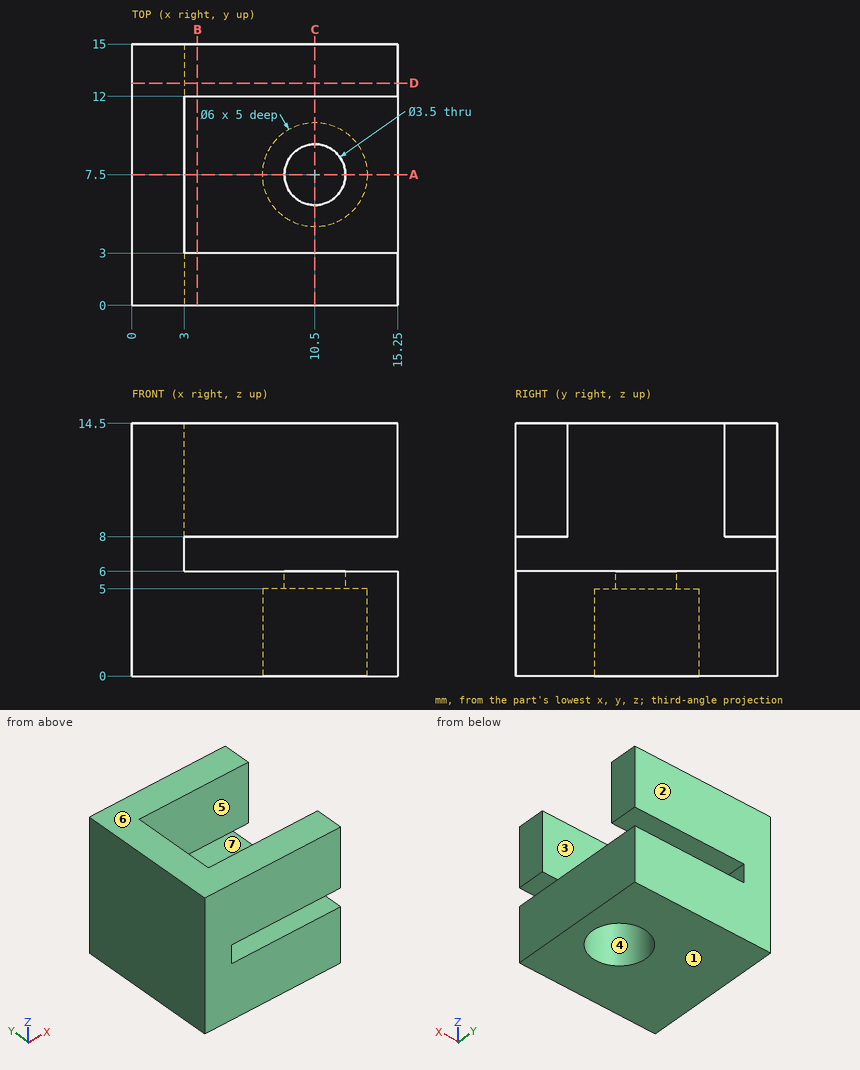
The drawing under review shows one solid part. Ordinate dimensions are in mm from its lowest x, y, z. A direction names the side the tool comes from. Coordinates: 2 decimals unless noted, no trailing zeros. Order: outer loops, then holes, each group sorted by start corner. A loop starts at its lowest first (then second) coordinate and runs counter-clockwise, first axis right, second up. Notation, with made-up numbers: (-17, 17.5) -> (35, 17.5) arc R26 ccw to (35, 32.5) -> close; hole circle Ø7 at (83.25, 85.5). An arc over 180 degrees is marked (long way). Return JSON: item names as keys, results as strings.
1. We need section A-A on y = 7.5. Write out the cut boundary in (x, z), and give its area (3 significant figures).
Answer block:
{"outline": "(0, 0) -> (7.5, 0) -> (7.5, 5) -> (8.75, 5) -> (8.75, 6) -> (3, 6) -> (3, 14.5) -> (0, 14.5) -> close; (12.25, 5) -> (13.5, 5) -> (13.5, 0) -> (15.25, 0) -> (15.25, 6) -> (12.25, 6) -> close", "area": "83.5 mm²"}
2. We need section D-D on y = 12.75. Write out the cut boundary in (x, z), and give its area (3 significant figures).
Answer block:
{"outline": "(0, 0) -> (15.25, 0) -> (15.25, 6) -> (3, 6) -> (3, 8) -> (15.25, 8) -> (15.25, 14.5) -> (0, 14.5) -> close", "area": "197 mm²"}
3. Machinability: for the marked faces 5, 6 and 7, which of the approach directions +Z, -Z, +X, -X, +Y, -Y give a long, thin tool a straight path to every point of the face, cutting with its end or side? Answer none if there is none.
Answer block:
{"face 5": "+Z, +X", "face 6": "+Z, +X, -X, +Y, -Y", "face 7": "+X, +Y, -Y"}
4. For pin 1 Ø5 at (x, y) = (5, 4) entering from -Z; pin 2 Ø7 at (x, y) = (10.5, 7.5) entering from +Z; pin 3 Ø2.5 at (y, z) = (6.5, 10) entering from +X, all flat-tipped, find the tip position at first contact; note any pin that passes through.
Answer block:
{"pin 1": "z = 0", "pin 2": "z = 6", "pin 3": "x = 3"}
5. The part is to be moulded in two halves that separate along Y. For the marked faces 1, 2, 3 and 4, say which applies: +Y half, -Y half, draft (parallel to the pull), parting line (faces both ways), or undercut.
Answer block:
{"face 1": "draft", "face 2": "+Y half", "face 3": "undercut", "face 4": "undercut"}
6. We need section B-B on x = 3.75. Write out the cut boundary in (y, z), and give its area (3 significant figures).
Answer block:
{"outline": "(0, 0) -> (15, 0) -> (15, 6) -> (0, 6) -> close; (0, 8) -> (3, 8) -> (3, 14.5) -> (0, 14.5) -> close; (12, 8) -> (15, 8) -> (15, 14.5) -> (12, 14.5) -> close", "area": "129 mm²"}
7. We need section C-C on x = 10.5. Write out the cut boundary in (y, z), and give its area (3 significant figures).
Answer block:
{"outline": "(0, 0) -> (4.5, 0) -> (4.5, 5) -> (5.75, 5) -> (5.75, 6) -> (0, 6) -> close; (0, 8) -> (3, 8) -> (3, 14.5) -> (0, 14.5) -> close; (9.25, 5) -> (10.5, 5) -> (10.5, 0) -> (15, 0) -> (15, 6) -> (9.25, 6) -> close; (12, 8) -> (15, 8) -> (15, 14.5) -> (12, 14.5) -> close", "area": "95.5 mm²"}
8. For line 1 (Z direction, x = 10, y = 2.25); line 2 (X direction, y = 7.5, z = 5.75); line 3 (X direction, y = 7.5, z = 2.6), list the stretches that pass through material, from the lowest coordinate up. Write a range as from..to.
Answer block:
{"line 1": "0..6, 8..14.5", "line 2": "0..8.75, 12.25..15.25", "line 3": "0..7.5, 13.5..15.25"}
